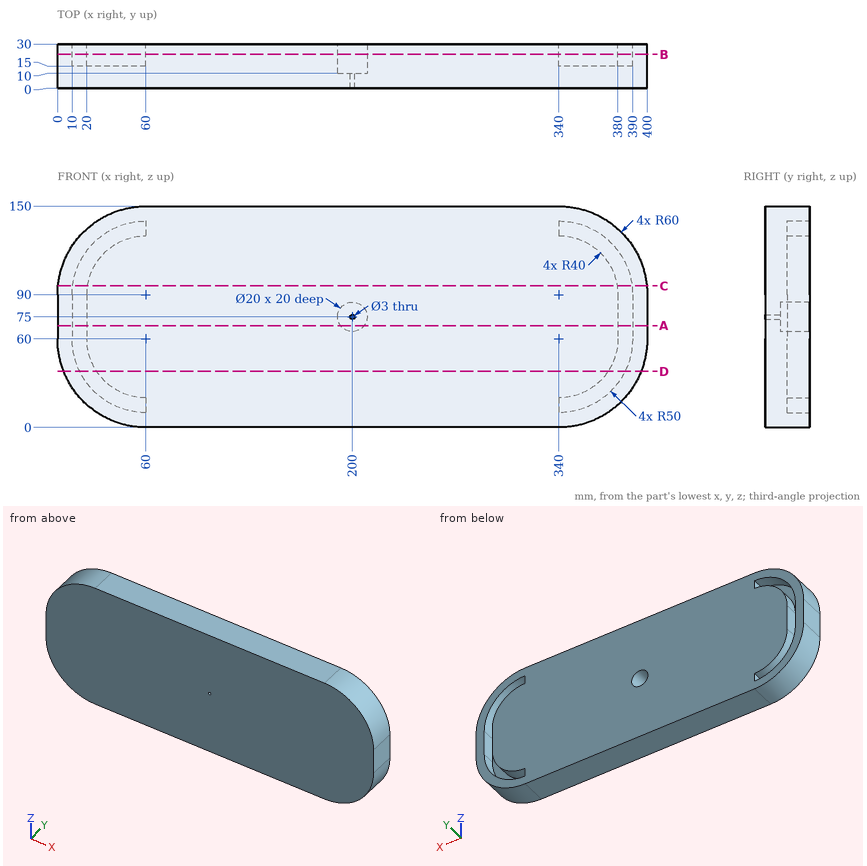
Check sheet for the drawn part. Datum: minimum x, y, z corner. Units: mm. Round coordinates to 2 decimals unless told otherwise and drop trailing zeros. Order: outer loops, then holes, each group sorted by start corner. A loop starts at its lowest first (then second) coordinate and runs counter-clockwise, first axis right, second up. Notation, with made-up numbers: M 44,-31.5 L 50,-31.5 A14 ccw 50,-4.5 Z; hole C 14,85.25 d1. An arc over 180 degrees is marked long. Write each question's results on one line, items separated by ' | '. Start each with the question number.
1. Material ranges on L1, parallel to Z at x = 38, y = 20; L2, parallel to X at y = 2.5, z = 75; L3, parallel to Z at x = 54, y = 21.5, recorded low to high. Write a range as from..to.
2. Cross-section at B-B on y = 23. Record the boundary of the cut face in (x, z), plus the area to 3 significant figures.
3. Cross-section at D-D on z = 38. Record the boundary of the cut face in (x, y).
4. Cross-section at C-C on z = 96. Record the boundary of the cut face in (x, y).
5. Go/stop test with flat-tipped pins: P1, Ø4, axis at x = 135.5, y = 19.5, coming from the -Z side; P2, Ø11, axis at y = 23, z = 137, coming from the +X side; P3, Ø16, axis at x = 200.5, z = 76.5, coming from the +Y side; P4, Ø8, axis at y = 23, z = 134, coming from the -X side. Record where each tip stops, or that it passes through.
6. Cross-section at A-A on z = 69. Record the boundary of the cut face in (x, y), plus the area to 3 significant figures.
Resolved:
1) L1: 4.18..15.1, 26.59..123.41, 134.9..145.82 | L2: 0..198.5, 201.5..400 | L3: 0.3..10.36, 20.45..129.55, 139.64..149.7
2) outline: M 0,60 A60 ccw 60,0 L 340,0 A60 ccw 400,60 L 400,90 A60 ccw 340,150 L 60,150 A60 ccw 0,90 Z; hole M 10,60 A50 ccw 60,10 L 60,20 A40 cw 20,60 L 20,90 A40 cw 60,130 L 60,140 A50 ccw 10,90 Z; hole C 200,75 d20; hole M 340,10 A50 ccw 390,60 L 390,90 A50 ccw 340,140 L 340,130 A40 cw 380,90 L 380,60 A40 cw 340,20 Z | area: 53,200 mm2
3) outline: M 4.18,0 L 395.82,0 L 395.82,30 L 384.9,30 L 384.9,15 L 373.41,15 L 373.41,30 L 26.59,30 L 26.59,15 L 15.1,15 L 15.1,30 L 4.18,30 Z
4) outline: M 0.3,0 L 399.7,0 L 399.7,30 L 389.64,30 L 389.64,15 L 379.55,15 L 379.55,30 L 20.45,30 L 20.45,15 L 10.36,15 L 10.36,30 L 0.3,30 Z
5) P1: z = 0 | P2: x = 383.33 | P3: y = 10 | P4: x = 15.28
6) outline: M 0,0 L 400,0 L 400,30 L 390,30 L 390,15 L 380,15 L 380,30 L 208,30 L 208,10 L 192,10 L 192,30 L 20,30 L 20,15 L 10,15 L 10,30 L 0,30 Z | area: 11,400 mm2
